For this review, use the dimensioned drawing (mm, ordinates from the lowest corner) and the shaded views. Round coordinates to 2 decimals unless told otherwise and drop trailing zeros. Write each loop counter-clockwise with the first axis right and the second up, starting at its lowest first coordinate (ties: lowest second). Pieces come first, ordered by that corner, then holes. Notation, with made-up numbers: M -11,39.5 L 43,39.5 A14 cw 43,55.5 Z; hole C -21.5,-38.75 d7. An arc over 180 degrees is marked long. Answer in a Markdown table with one row per item.
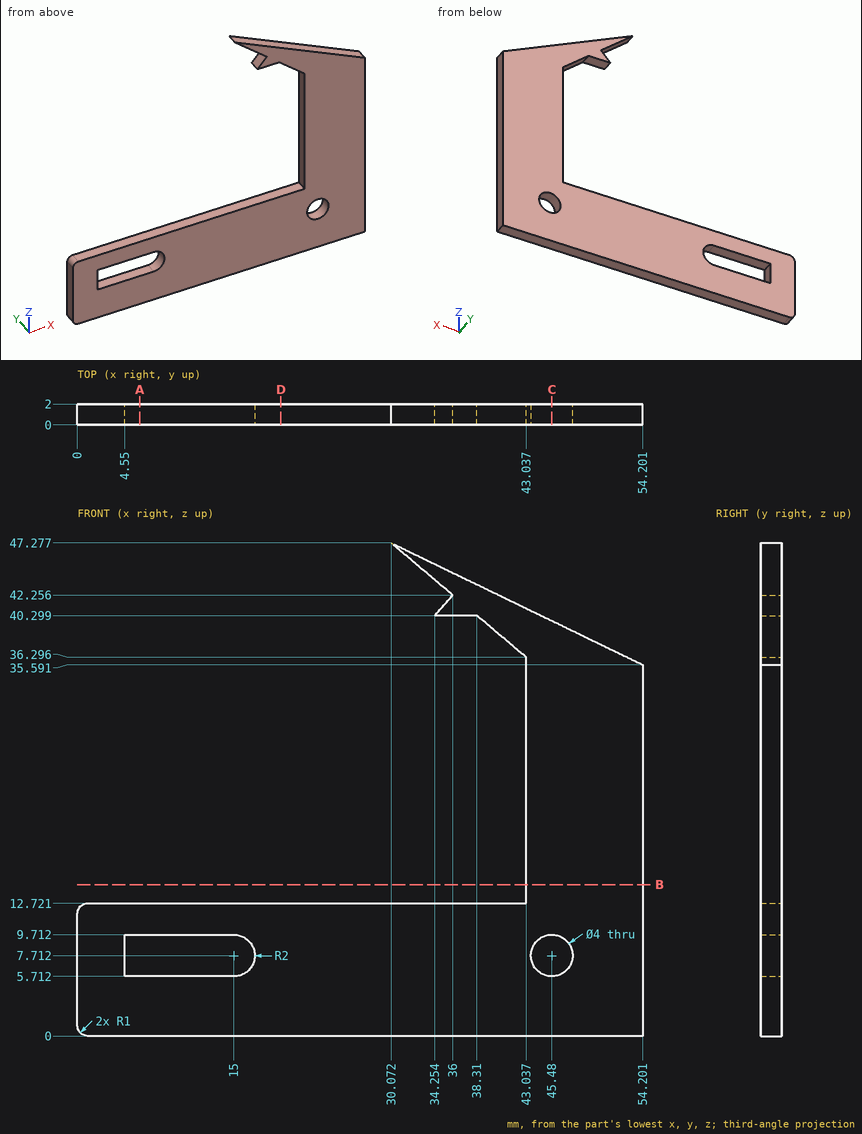
Q1. For probe 1 along X at (y, z) = (0.2, 7.5); probe 2 along Z at (x, y) = (9, 1.9); probe 3 along X at (y, z) = (0.55, 26), list the stretches that pass through material, from the lowest coordinate up.
Found:
| item | result |
|---|---|
| probe 1 | 0 to 4.55, 16.99 to 43.49, 47.47 to 54.2 |
| probe 2 | 0 to 5.71, 9.71 to 12.72 |
| probe 3 | 43.04 to 54.2 |
Q2. Take a section at B-B (z = 14.5). State the section outline as (x, y) points.
Found:
| item | result |
|---|---|
| outline | M 43.04,0 L 54.2,0 L 54.2,2 L 43.04,2 Z |
Q3. Take a section at A-A (x = 6). State the section outline as (y, z) points.
Found:
| item | result |
|---|---|
| outline | M 0,0 L 2,0 L 2,5.71 L 0,5.71 Z; M 0,9.71 L 2,9.71 L 2,12.72 L 0,12.72 Z |
Q4. Insertion check: P1, Ø5, axis at x = 45.48, z = 7.71, coming from the -Y side; P2, Ø1, axis at y = 1, z = 27.5, coming from the -X side. Each pin has a flat end and moves straight along its axis. Give the tip position at first contact, or say it passes through.
Found:
| item | result |
|---|---|
| P1 | y = 0 |
| P2 | x = 43.04 |
Q5. Take a section at C-C (x = 45.48). State the section outline as (y, z) points (1 decimal).
Found:
| item | result |
|---|---|
| outline | M 0,0 L 2,0 L 2,5.7 L 0,5.7 Z; M 0,9.7 L 2,9.7 L 2,39.8 L 0,39.8 Z |
Q6. Take a section at D-D (x = 19.5). State the section outline as (y, z) points.
Found:
| item | result |
|---|---|
| outline | M 0,0 L 2,0 L 2,12.72 L 0,12.72 Z |
